Study the drawing (mm; zero at the part's minimum x, y, z) and answer. A direction names the side the tool comes from. Give positions to 0.01 mm unless a question says otherwise; leave off trailing zeros. Loops run counter-clockwise (first coordinate to the right, second up) from the corner with the lowest first, then second, coordinate; pieces in that order, holes last. Notation, with made-up numbers: (50.5, -22.5) - (85.5, -22.5) arc R17 ccw to (85.5, -11.5) - close; hole circle Ø2 at (84.5, 38). An arc over 180 degrees is marked (long way). Use one line per item in the form item = value. Start each with the question number.
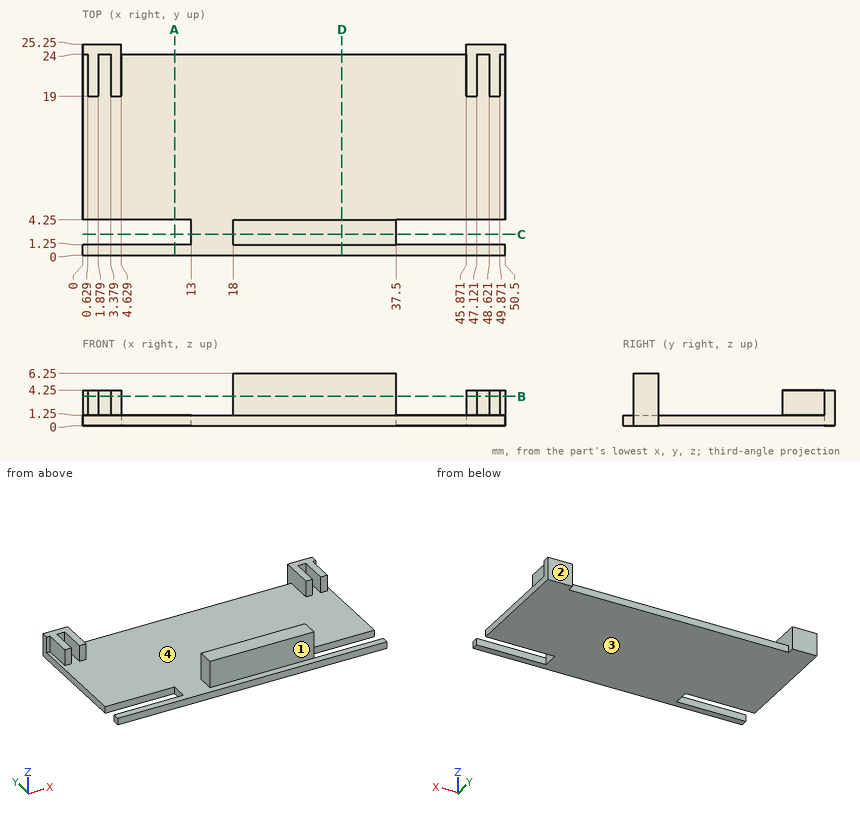
1) A cutting plane is placed at D-D (x = 31). Give the vertices of the cut face in (y, z).
2) Determine the mould class of the marked faces 3 and 4 for opening direction X: released by +X, released by -X, zero draft, split by the parting line, or undercut.
3) A cutting plane is placed at C-C (y = 2.5). Give the vertices of the cut face in (x, z).
4) A cutting plane is placed at B-B (z = 3.5). Give the vertices of the cut face in (x, y).
5) A cutting plane is placed at A-A (x = 11). Give the vertices of the cut face in (y, z).
6) Flat-ended cylindrical pins translate along their axes: pin 1 Ø1.4 at (x, z) = (46.5, 2.5) entering from -Y; pin 2 Ø1.5 at (y, z) = (3, 4) entering from -X; pin 3 Ø2 at (x, z) = (30, 2) entering from +Y. Find the tip coordinate at first contact, or state that the pin passes through.
7) Find the intervals of material crossed by probe 1 along X at (y, z) = (23.5, 2); probe 2 along X at (y, z) = (24.25, 3); probe 3 along X at (y, z) = (2.5, 5.25), in increasing order.
8) A tool of negligible diameter and unlimited length cuts with its end or side. For the marked faces 1 and 2, from which of +Z, -Z, +X, -X, +Y, -Y can it reach the whole face along a straight path? Write none if from no direction.
Answer sheet:
q1.outline = (0, 0) - (24, 0) - (24, 1.25) - (4.25, 1.25) - (4.25, 6.25) - (1.25, 6.25) - (1.25, 1.25) - (0, 1.25) - close
q2.face_3 = zero draft
q2.face_4 = undercut
q3.outline = (13, 0) - (37.5, 0) - (37.5, 6.25) - (18, 6.25) - (18, 1.25) - (13, 1.25) - close
q4.outline = (0, 24) - (0.63, 24) - (0.63, 19) - (1.88, 19) - (1.88, 24) - (3.38, 24) - (3.38, 19) - (4.63, 19) - (4.63, 25.25) - (0, 25.25) - close; (18, 1.25) - (37.5, 1.25) - (37.5, 4.25) - (18, 4.25) - close; (45.87, 19) - (47.12, 19) - (47.12, 24) - (48.62, 24) - (48.62, 19) - (49.87, 19) - (49.87, 24) - (50.5, 24) - (50.5, 25.25) - (45.87, 25.25) - close
q5.outline = (0, 0) - (1.25, 0) - (1.25, 1.25) - (0, 1.25) - close; (4.25, 0) - (24, 0) - (24, 1.25) - (4.25, 1.25) - close
q6.pin_1 = 19
q6.pin_2 = 18
q6.pin_3 = 24
q7.probe_1 = 0.63 to 1.88, 3.38 to 4.63, 45.87 to 47.12, 48.62 to 49.87
q7.probe_2 = 0 to 4.63, 45.87 to 50.5
q7.probe_3 = 18 to 37.5
q8.face_1 = +Z, +X, -X, -Y
q8.face_2 = +Z, -Z, +X, -X, +Y
